from build123d import *

# Parameters (mm, degrees)
BOSS_EXTRUDE1_DEPTH = 3
BOSS_EXTRUDE2_DEPTH = 41.8
SKETCH5_R           = 2.6
CUT_EXTRUDE1_DEPTH  = 0.6


with BuildPart() as part:
    # Sketch2 → Boss-Extrude1 (new body)
    with BuildSketch(Plane(origin=(0, 0, 0), x_dir=(1, 0, 0), z_dir=(0, 1, 0))):
        with BuildLine():
            Line((-20.9, 1.4), (-20.9, 14.9))
            Line((-20.9, 14.9), (20.9, 14.9))
            Line((20.9, 14.9), (20.9, -14.9))
            Line((20.9, -14.9), (-20.9, -14.9))
            Line((-20.9, -14.9), (-20.9, -1.4))
            ThreePointArc((-20.9, -1.4), (-19.5, 0), (-20.9, 1.4))
        make_face()
    extrude(amount=BOSS_EXTRUDE1_DEPTH)

    # Sketch4 → Boss-Extrude2 (add)
    with BuildSketch(Plane.ZY.offset(20.9)):
        Polygon((-14.9, 3), (-14.9, 4.8), (-16.9, 6.8), (-14.9, 8.8), (-14.9, 10), (-11.9, 10), (-11.9, 3), align=None)
        Polygon((14.9, 3), (11.9, 3), (11.9, 10), (14.9, 10), (14.9, 8.8), (16.9, 6.8), (14.9, 4.8), align=None)
    extrude(amount=-BOSS_EXTRUDE2_DEPTH)

    # Sketch5 → Cut-Extrude1 (cut)
    with BuildSketch(Plane.XZ):
        with Locations(Location((0, 0, 0), (0, 0, 270))):
            Circle(SKETCH5_R)
    extrude(amount=-CUT_EXTRUDE1_DEPTH, mode=Mode.SUBTRACT)


solid = part.part
The listing builds one solid part. Answer for the finished solid, in the listing's coordinates (mm). A direction names the side the tool comes from. Give positions to 0.01 mm unless a question says otherwise; leave off trailing zeros. Write each loop counter-clockwise with the first axis right and the second up, starting at its lowest first coordinate (ties: lowest second). Pieces come first, ordered by that corner, then holes.
Item 1: Section A-A, the plane y = 5.75 is taken. Write down the section's boundary in (x, z).
Item 2: Find the intervals of material crossed by line 1 along X through (y, z) = (0.3, 0); line 2 along Z through (x, y) = (-5.5, 4); line 3 along Y through (x, z) = (13.5, -3.5), in increasing order.
Item 3: Flat-ended cylindrical pins translate along their axes: P1, Ø1.6, axis at x = 0, z = -1, coming from the -Y side; P2, Ø5.5, axis at x = 9, y = 7, coming from the -Z side; P3, Ø4, axis at x = 3, y = 2.5, coming from the +Z side; P4, Ø6, axis at x = -9, y = 8.5, coming from the +Z side. Find the tip coordinate at first contact, or state that the pin passes through.
Item 4: Section D-D, the plane x = 0 is taken. Write down the section's boundary in (y, z).
Item 5: Which of the six approach directions +Z, -Z, +X, -X, +Y, -Y give full straight-line access (tool end or side, diameter ignored) to faces 1 (the cylindrical face through (0.78, 0.3, -2.48)), 2 (the flat face through (0, 9, -14.9)), 3 (the flat face through (0, 9, 14.9)), 4 (the flat face through (0, 7, -11.9)), 5 (the flat face through (0, 2, -14.9))?
Item 6: Determine the mould class of faces 6 (the cylindrical face through (-19.5, 1.5, 0)), 7 (the flat face through (0, 10, 13)), 8 (the flat face through (0, 2, 14.9)) for opening direction Z: released by +Z, released by -Z, zero draft, split by the parting line, or undercut.
Item 7: Section B-B, the plane z = 0 is taken. Write down the section's boundary in (x, y), plus the area to 3 significant figures.
Item 8: Section C-C, the plane x = -16.5 is taken. Write down the section's boundary in (y, z), plus the area to 3 significant figures.
Completed:
1. outline: (-20.9, -15.85) - (20.9, -15.85) - (20.9, -11.9) - (-20.9, -11.9) - close; (-20.9, 11.9) - (20.9, 11.9) - (20.9, 15.85) - (-20.9, 15.85) - close
2. line 1: x = -19.5 to -2.6, 2.6 to 20.9
2. line 2: z = -14.9 to -11.9, 11.9 to 14.9
2. line 3: y = 0 to 3
3. P1: stops at y = 0.6
3. P2: stops at z = -16.9
3. P3: stops at z = 14.9
3. P4: stops at z = 16.9
4. outline: (0, -14.9) - (4.8, -14.9) - (6.8, -16.9) - (8.8, -14.9) - (10, -14.9) - (10, -11.9) - (3, -11.9) - (3, 11.9) - (10, 11.9) - (10, 14.9) - (8.8, 14.9) - (6.8, 16.9) - (4.8, 14.9) - (0, 14.9) - (0, 2.6) - (0.6, 2.6) - (0.6, -2.6) - (0, -2.6) - close
5. face 1: -Y
5. face 2: -Z, +X, -X, +Y
5. face 3: +Z, +X, -X, +Y
5. face 4: +X, -X, +Y
5. face 5: -Z, +X, -X, -Y
6. face 6: undercut
6. face 7: zero draft
6. face 8: released by +Z
7. outline: (-19.5, 0) - (-2.6, 0) - (-2.6, 0.6) - (2.6, 0.6) - (2.6, 0) - (20.9, 0) - (20.9, 3) - (-19.5, 3) - close
7. area: 118 mm2
8. outline: (0, -14.9) - (4.8, -14.9) - (6.8, -16.9) - (8.8, -14.9) - (10, -14.9) - (10, -11.9) - (3, -11.9) - (3, 11.9) - (10, 11.9) - (10, 14.9) - (8.8, 14.9) - (6.8, 16.9) - (4.8, 14.9) - (0, 14.9) - close
8. area: 139 mm2
